Autodesk Inventor part; units mm, degrees
ref_plane "YZ Plane" through (0, 0, 0) normal (1, 0, 0) x (0, 1, 0)
ref_plane "XZ Plane" through (0, 0, 0) normal (0, 1, 0) x (-1, 0, 0)
ref_plane "XY Plane" through (0, 0, 0) normal (0, 0, 1) x (1, 0, 0)
sketch "スケッチ1" plane through (0, 0, 0) normal (0, 1, 0) x (-1, 0, 0)
  line L0 (12.5, 22.5) -> (-12.5, 22.5)
  line L1 (-12.5, 22.5) -> (-12.5, -22.5)
  line L2 (-12.5, -22.5) -> (12.5, -22.5)
  line L3 (12.5, -22.5) -> (12.5, 22.5)
  line L4 (12.5, 22.5) -> (-12.5, -22.5) construction
  line L5 (-12.5, 22.5) -> (12.5, -22.5) construction
  line L6 (12.5, 22.5) -> (12.5, 27.5)
  line L7 (12.5, 27.5) -> (-12.5, 27.5)
  line L8 (-12.5, 27.5) -> (-12.5, 22.5)
  point P0 (0, 0)
  dimension "d0" = 45
  dimension "d2" = 25
  dimension "d3" = 5
extrude "押し出し1" add sketch "スケッチ1" along normal blind 2
sketch "スケッチ2" plane through (0, 2, 0) normal (0, 1, 0) x (1, 0, 0)
  line L0 (-12.5, -27.5) -> (12.5, -27.5) construction
  line L1 (12.5, -27.5) -> (12.5, 22.5) construction
  line L2 (12.5, 22.5) -> (-12.5, 22.5) construction
  line L3 (-12.5, 22.5) -> (-12.5, -27.5) construction
  line L4 (0, 32.5) -> (0, -37.5) construction
  line L5 (-12.5, -27.5) -> (12.5, -27.5)
  line L6 (12.5, -27.5) -> (12.5, 22.5)
  line L7 (12.5, 22.5) -> (-12.5, 22.5)
  line L8 (-12.5, 22.5) -> (-12.5, -27.5)
  line L9 (-12.5, 22.5) -> (-12.5, -27.5)
  line L10 (12.5, 22.5) -> (-12.5, 22.5)
  point P0 (0, 0)
  point P1 (0, -27.5)
extrude "押し出し2" add sketch "スケッチ2" along normal blind 2
sketch "スケッチ3" plane through (0, 4, 0) normal (0, 1, 0) x (1, 0, 0)
  line L0 (-12.5, 22.5) -> (-12.5, -2) construction
  line L1 (-12.5, -2) -> (12.5, -2) construction
  line L2 (12.5, -2) -> (12.5, 22.5) construction
  line L3 (12.5, 22.5) -> (-12.5, 22.5) construction
  line L4 (-12.5, 22.5) -> (-12.5, -2) construction
  line L5 (-12.5, -27.5) -> (12.5, -27.5)
  line L6 (12.5, -27.5) -> (12.5, 22.5)
  line L7 (12.5, 22.5) -> (-12.5, 22.5)
  line L8 (-12.5, 22.5) -> (-12.5, -27.5)
  line L9 (-12.5, -27.5) -> (12.5, -27.5) construction
  point P0 (0, 0)
extrude "押し出し3" add sketch "スケッチ3" along normal blind 8
sketch "スケッチ4" plane through (0, 12, 0) normal (0, 1, 0) x (1, 0, 0)
  line L0 (12.5, -2) -> (12.5, 22.5) construction
  line L1 (-5.5, 22.5) -> (5.5, 22.5)
  line L2 (5.5, 22.5) -> (5.5, -23.5)
  line L3 (5.5, -23.5) -> (-5.5, -23.5)
  line L4 (-5.5, -23.5) -> (-5.5, 22.5)
  line L5 (0, 32.5) -> (0, -37.5) construction
  circle A0 centre (0, -18.4) radius 1.5
  circle A1 centre (0, -11) radius 1.5
  line L6 (-17.5, 0) -> (17.5, 0) construction
  line L7 (-5.5, -6.9) -> (5.5, -6.9)
  line L8 (12.5, -27.5) -> (12.5, 22.5) construction
  line L9 (12.5, 22.5) -> (-12.5, 22.5) construction
  line L10 (-12.5, 22.5) -> (-12.5, -27.5) construction
  line L11 (-12.5, -27.5) -> (12.5, -27.5) construction
  line L12 (12.5, 22.5) -> (-12.5, 22.5)
  point P0 (0, 0)
  point P1 (0, -23.5)
  dimension "d14" = 11
  dimension "d15" = 3
  dimension "d16" = 7.4
  dimension "d17" = 22
  dimension "d24" = 16.6
  dimension "d27" = 46
extrude "押し出し4" cut sketch "スケッチ4" against normal blind 8 contours L1 L2 L7 L4 | L7 L2 L3 L4 | A0 | A1
extrude "押し出し5" cut sketch "スケッチ4" against normal through all contours A0 | A1
extrude "押し出し6" cut sketch "スケッチ4" against normal blind 10 contours L1 L2 L7 L4
sketch "スケッチ5" plane through (0, 0, 0) normal (0, -1, 0) x (1, 0, 0)
  circle A0 centre (0, 18.4) radius 1.5 construction
  circle A1 centre (0, 11) radius 1.5 construction
  circle A2 centre (0, 18.4) radius 2.75
  circle A3 centre (0, 11) radius 2.75
  point P0 (0, 0)
  dimension "d28" = 5.5
extrude "押し出し7" cut sketch "スケッチ5" against normal blind 2.5
fillet "フィレット1" radius 6 6 edges at (12.5, 0, 2.5) (-12.5, 0, 2.5) (0, 0, 27.5) (12.5, 6, 27.5) (-12.5, 6, 27.5) (0, 0, -22.5)
sketch "スケッチ6" plane through (0, 0, 0) normal (1, 0, 0) x (0, 1, 0)
  line L0 (12, 23.5) -> (12, -22.5) construction
  line L1 (12, -22.5) -> (2, -22.5) construction
  line L2 (12, -22.5) -> (6, -22.5)
  line L3 (6, -22.5) -> (6, -4.5)
  line L4 (6, -4.5) -> (12, -4.5)
  line L5 (12, -4.5) -> (12, -22.5)
  point P0 (0, 0)
  dimension "d32" = 6
  dimension "d33" = 18
extrude "押し出し8" cut sketch "スケッチ6" along normal through all both and the other way through all
sketch "スケッチ7" plane through (0, 12, 0) normal (0, 1, 0) x (1, 0, 0)
  line L0 (5.5, -6.9) -> (-5.5, -6.9)
  line L1 (-28.6346, -6.9) -> (35.9523, -6.9)
  line L2 (35.9523, -6.9) -> (35.9523, 63.9707)
  line L3 (35.9523, 63.9707) -> (-28.6346, 63.9707)
  line L4 (-28.6346, 63.9707) -> (-28.6346, -6.9)
  point P0 (0, 0)
properties part number "pressure_plate" material "ABS プラスチック"
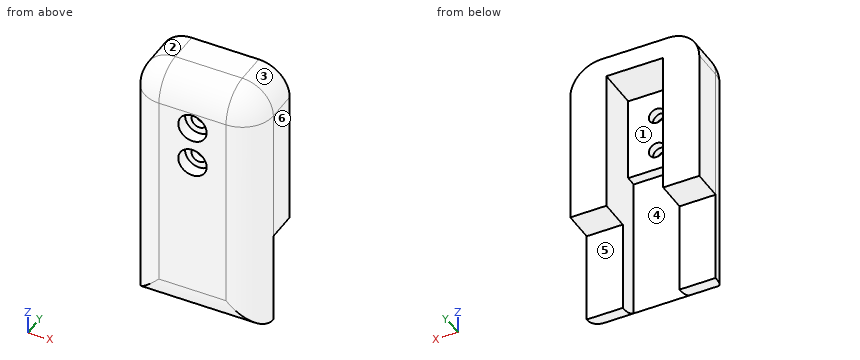
Can you work these out from the model? Positions are in its coordinate system, mm. Face numbers are marked on the shaded views. A direction names the side the tool comes from. Coordinates: 2 decimals unless noted, no trailing zeros. Loops run counter-clockwise (first coordinate to the right, second up) from the corner with the lowest first, then second, coordinate; pieces in that order, holes last. Notation, with made-up numbers: (-25.5, 52.25) -> (-0.5, 52.25) arc R34 ccw to (-0.5, 88.25) -> close; hole circle Ø9 at (-34, 53). An arc over 180 degrees is marked (long way). Put each result on its own line as item: value. Start each with the question number.
Q1. I'm going to push flat-ended pins straight in: P1, Ø7.5, axis at x = -8, z = -17, coming from the +Y side; P2, Ø3, axis at x = 9.5, y = 8, coming from the -Z side; P3, Ø4, axis at x = 2, y = 7.5, coming from the -Z side. Where does each tip first touch, or does it pass through?
Q2. If I drill on line 1 (Z direction, x = 0, y = 2.8); line 2 (X direction, y = 6.75, z = 1.5); line 3 (Z direction, x = 0, y = 1.55), over which ranges is the centre line in solid material (lowest first)? Write a range as [from, to].
Q3. For the marked faces 4, 5 and 6, which set-ups out of +Z, -Z, +X, -X, +Y, -Y let a thin tool reach every point of the face, with its end or its side?
Q4. I want a section at A-A (z = 11). Write out the boundary of the cut face in (x, y).
Q5. I want a section at D-D (y = 9). Write out the boundary of the cut face in (x, z), plus the area to 3 significant figures.
Q6. I want a section at C-C (x = -5). Write out the boundary of the cut face in (y, z).
Q7. Thinking about a two-plate mould opening in X: for the marked faces 1, 2 and 3, which applies, pulls with the +X half, pulls with the -X half, needs draft (parallel to the pull), parting line crosses it, or undercut?
Q8. I want a section at B-B (x = 0). Write out the boundary of the cut face in (y, z).
Taken from the geometry:
1. P1: stops at y = 6
1. P2: stops at z = -4.5
1. P3: stops at z = 23.5
2. line 1: z = [6.9, 9.5], [12.5, 16.9], [19.9, 26.58]
2. line 2: x = [-12.5, -5.5], [5.5, 12.5]
2. line 3: z = [-20.52, 8.25], [13.75, 15.65], [21.15, 25.52]
3. face 4: -Z, +Y
3. face 5: -Z, +X, -X, +Y
3. face 6: +Z, -Z, +X, +Y, -Y
4. outline: (-12.5, 6) arc R6 ccw to (-6.5, 0) -> (-2.75, 0) -> (-2.75, 2.5) -> (-1.5, 2.5) -> (-1.5, 4) -> (-5.5, 4) -> (-5.5, 12) -> (-12.5, 12) -> close; (1.5, 2.5) -> (2.75, 2.5) -> (2.75, 0) -> (6.5, 0) arc R6 ccw to (12.5, 6) -> (12.5, 12) -> (5.5, 12) -> (5.5, 4) -> (1.5, 4) -> close
5. outline: (-12.5, -4.5) -> (-5.5, -4.5) -> (-5.5, 23.5) -> (5.5, 23.5) -> (5.5, -4.5) -> (12.5, -4.5) -> (12.5, 21.5) arc R6 ccw to (6.5, 27.5) -> (-6.5, 27.5) arc R6 ccw to (-12.5, 21.5) -> close
5. area: 477 mm2
6. outline: (0, -16.5) arc R6 ccw to (2, -20.97) -> (2, 6.9) -> (4, 6.9) -> (4, 23.5) -> (12, 23.5) -> (12, 27.5) -> (6, 27.5) arc R6 ccw to (0, 21.5) -> close
7. face 1: undercut
7. face 2: pulls with the -X half
7. face 3: pulls with the +X half
8. outline: (0, -16.5) arc R6 ccw to (2, -20.97) -> (2, 6.9) -> (4, 6.9) -> (4, 9.5) -> (2.5, 9.5) -> (2.5, 8.25) -> (0, 8.25) -> close; (0, 13.75) -> (2.5, 13.75) -> (2.5, 12.5) -> (4, 12.5) -> (4, 16.9) -> (2.5, 16.9) -> (2.5, 15.65) -> (0, 15.65) -> close; (0, 21.15) -> (2.5, 21.15) -> (2.5, 19.9) -> (4, 19.9) -> (4, 23.5) -> (12, 23.5) -> (12, 27.5) -> (6, 27.5) arc R6 ccw to (0, 21.5) -> close
